Answer from the drawing. Dimensions are ordinates in mm from the lowest x, y and z of the part. A direction names the side the tool comes from. Give positions to 0.01 mm unless a question says otherwise; leave off trailing zeros. Write each loop counter-clockwise with the first axis right and the second up, starting at its lowest first coordinate (ties: lowest second). Pieces come first, ordered by that corner, then holes. Notation, with made-up numbers: M -28,59 L -24,59 A14 cw -24,64 Z; hole C 45,8.25 d5. An arc over 180 degrees is marked long. Answer as a JSON object with one key per item and string values.
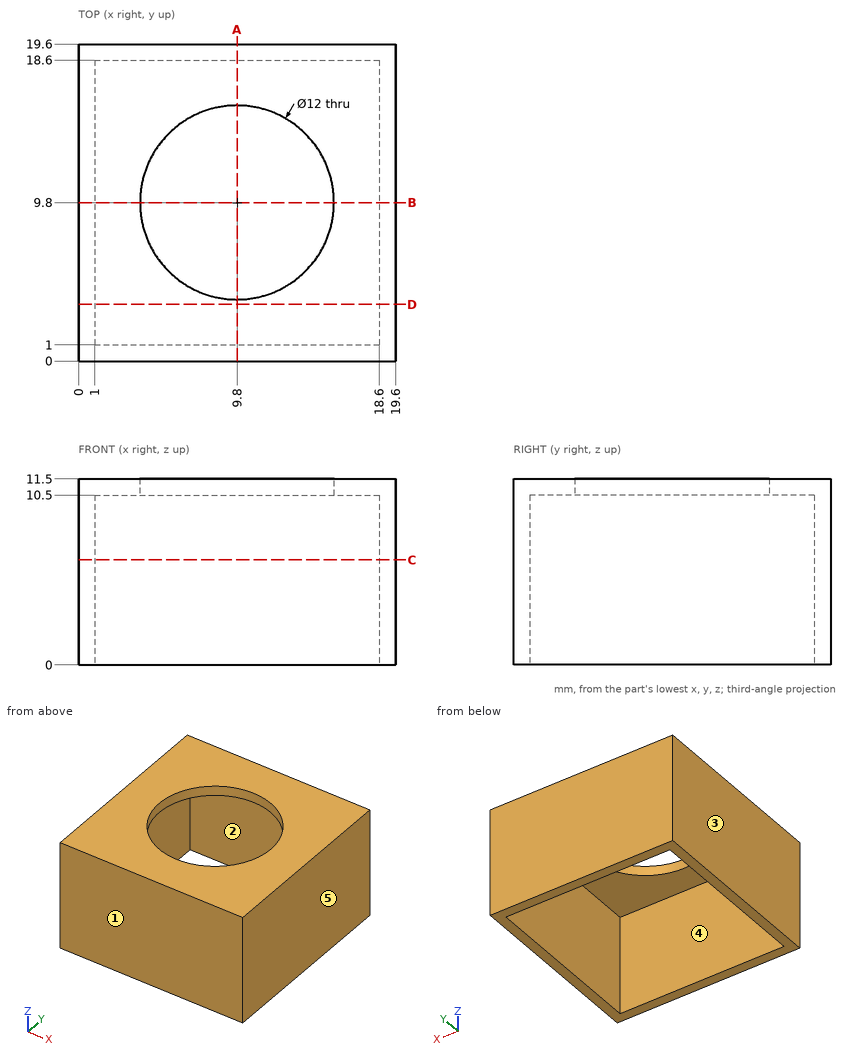
1. A cutting plane is placed at C-C, the plane z = 6.5. Give the vertices of the cut face in (x, y), plus the area to 3 significant figures.
Verdict:
{"outline": "M 0,0 L 19.6,0 L 19.6,19.6 L 0,19.6 Z; hole M 1,1 L 18.6,1 L 18.6,18.6 L 1,18.6 Z", "area": "74.4 mm2"}
2. Consider line 1 along Y through (x, z) = (15.75, 6.75); line 2 along Y through (x, z) = (9.8, 10.8). Determine where each line is inside the solid, lowest interval first.
Verdict:
{"line 1": "y = 0 to 1, 18.6 to 19.6", "line 2": "y = 0 to 3.8, 15.8 to 19.6"}
3. A cutting plane is placed at D-D, the plane y = 3.5. Give the vertices of the cut face in (x, z), plus the area to 3 significant figures.
Verdict:
{"outline": "M 0,0 L 1,0 L 1,10.5 L 18.6,10.5 L 18.6,0 L 19.6,0 L 19.6,11.5 L 0,11.5 Z", "area": "40.6 mm2"}
4. A cutting plane is placed at A-A, the plane x = 9.8. Give the vertices of the cut face in (y, z), plus the area to 3 significant figures.
Verdict:
{"outline": "M 0,0 L 1,0 L 1,10.5 L 3.8,10.5 L 3.8,11.5 L 0,11.5 Z; M 15.8,10.5 L 18.6,10.5 L 18.6,0 L 19.6,0 L 19.6,11.5 L 15.8,11.5 Z", "area": "28.6 mm2"}
5. The mould has two halves that part along X. Classify the marked faces 1, 2 and 3: released by +X, released by -X, zero draft, split by the parting line, or undercut.
Verdict:
{"face 1": "zero draft", "face 2": "undercut", "face 3": "released by -X"}
6. For the marked faces 4 and 5, determine the directions among +Z, -Z, +X, -X, +Y, -Y from which every point of the face is accessible in a straight line to the end or side of a thin tool.
Verdict:
{"face 4": "-Z", "face 5": "+Z, -Z, +X, +Y, -Y"}
